Input: part model. Units: mm. Frame: model coordinates. A direction names the side the tool comes from. Coordinates: 2 decimals unless noted, no trailing zeros. Loops run counter-clockwise (first coordinate to the right, second up) from the corner with the lowest first, then second, coordinate; pieces in that order, holes last. Notation, with made-up numbers: (61, 36.25) - (68, 36.25) arc R16 cw to (68, 57.25) - close; hole circle Ø9 at (-40, -39.5). An arc over 180 degrees is marked (long way). Use one line per item in the form item = value.
Autodesk Fusion 360 part; units mm, degrees
sketch "Sketch1" plane through (0, 0, 0) normal (0, 1, 0) x (1, 0, 0)
  circle A0 centre (0, 0) radius 6.35
  dimension "d1" = 12.7
extrude "Extrude1" add sketch "Sketch1" along normal blind 5.5
sketch "Sketch2" plane through (0, 0, 0) normal (0, -1, 0) x (1, 0, 0)
  circle A0 centre (0, 0) radius 6.35
  circle A1 centre (0, 0) radius 9
  dimension "d4" = 18
extrude "Extrude2" add sketch "Sketch2" along normal blind 3 contours A0 | A1
sketch "Sketch3" plane through (0, -3, 0) normal (0, -1, 0) x (1, 0, 0)
  circle A0 centre (0, 0) radius 9
  circle A1 centre (0, 0) radius 2
  dimension "d7" = 4
hole "Hole1" at (0, -3, 0) direction (0, 1, 0) diameter 4.3 end through all counterbore diameter 8 counterbore depth 4
equation "d1 = 0'- 1/2\""
Q1. Ray query, line 1 along Z through (x, y) = (0, -0.3); line 2 along Z through (x, y) = (0, 2.05). Return the intervals inside material, ascending. Write a range as [from, to].
Check values:
line_1 = [-9, -4], [4, 9]
line_2 = [-6.35, -2.15], [2.15, 6.35]
Q2. Cut plane C-C, the plane y = 0.75. Return loops of the section in (x, z), then the cut area to 3 significant figures.
Check values:
outline = circle Ø12.7 at (0, 0); hole circle Ø8 at (0, 0)
area = 76.4 mm²
Q3. Cut plane A-A, the plane x = 0. Return loops of the section in (y, z), then the cut area to 3 significant figures.
Check values:
outline = (-3, -9) - (0, -9) - (0, -6.35) - (5.5, -6.35) - (5.5, -2.15) - (1, -2.15) - (1, -4) - (-3, -4) - close; (-3, 4) - (1, 4) - (1, 2.15) - (5.5, 2.15) - (5.5, 6.35) - (0, 6.35) - (0, 9) - (-3, 9) - close
area = 72.5 mm²
Q4. First-contact query: P1, Ø4, axis at y = 4, z = -5, coming from the +X side; P2, Ø7, axis at x = 0, z = 0, coming from the -Y side; P3, Ø2, axis at x = -3, y = 3.5, coming from the +Z side. Flat tips, straight axial feed; report the tip coordinate or a pass-through.
Check values:
P1 = 5.6
P2 = 1
P3 = 6.03
Q5. Pull-direction query (X, two-part tool) for faces 1 (the flat face through (4, 0, -6)), 2 (the cylindrical face through (3.905, -0.972, 0.867)), 3 (the cylindrical face through (-1.172, -1.479, -8.923)); classes: pulls with the +X half, pulls with the -X half, needs draft (parallel to the pull), parting line crosses it, or undercut.
Check values:
face_1 = needs draft
face_2 = undercut
face_3 = parting line crosses it
Q6. Set-up query: faces 4 (the flat face through (2, 1, -2)), 5 (the cylindrical face through (-1.38, 2.71, -6.2)), 6 (the cylindrical face through (-0.09, 3.28, 2.15)). Return all of +Z, -Z, +X, -X, +Y, -Y with unobstructed straight access to the full face (end or side cutting, diameter ignored); none if empty.
Check values:
face_4 = -Y
face_5 = +Y
face_6 = +Y, -Y
Q7. Cut plane B-B, the plane z = 0. Return loops of the section in (x, y).
Check values:
outline = (-9, -3) - (-4, -3) - (-4, 1) - (-2.15, 1) - (-2.15, 5.5) - (-6.35, 5.5) - (-6.35, 0) - (-9, 0) - close; (2.15, 1) - (4, 1) - (4, -3) - (9, -3) - (9, 0) - (6.35, 0) - (6.35, 5.5) - (2.15, 5.5) - close
Q8. Cut plane D-D, the plane x = 3.5. Return loops of the section in (y, z).
Check values:
outline = (-3, -8.29) - (0, -8.29) - (0, -5.3) - (5.5, -5.3) - (5.5, 5.3) - (0, 5.3) - (0, 8.29) - (-3, 8.29) - (-3, 1.94) - (1, 1.94) - (1, -1.94) - (-3, -1.94) - close
